Work out the finished part from the listing and answer in its coordinate system (mm). Round coordinates to 2 decimals unless told otherwise and drop trailing zeros. Loops run counter-clockwise (first coordinate to the right, second up) from the corner with the lowest first, then second, coordinate; pieces in that order, holes last. Notation, with made-up numbers: (5, 4.5) - (39, 4.5) arc R16 ccw to (39, 26.5) - close; hole circle Ø10 at (78.25, -4). An arc over 180 degrees is marked (long way). Return JSON: item names as keys, results as strings.
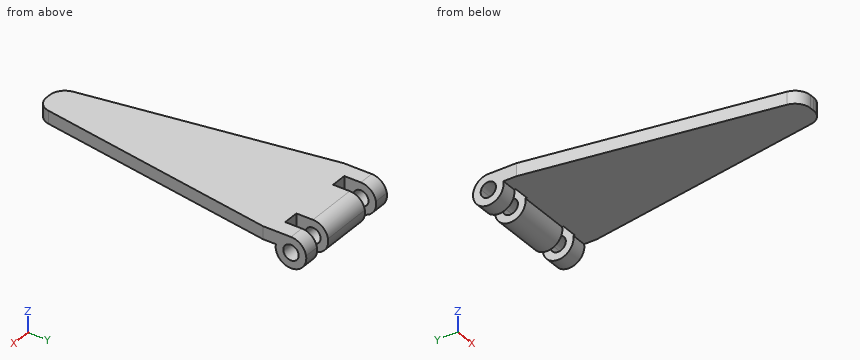
from build123d import *

# Parameters (mm, degrees)
CROQUIS1_W              = 45
CROQUIS1_H              = 17
SALIENTE_EXTRUIR1_DEPTH = 5
CROQUIS2_R              = 6
CROQUIS2_R_2            = 3
SALIENTE_EXTRUIR2_DEPTH = 45
CORTAR_EXTRUIR1_DEPTH   = 47.32763754
CROQUIS4_W              = 6.2
CROQUIS4_H              = 6.5
CROQUIS4_H_2            = 6
CORTAR_EXTRUIR2_DEPTH   = 27.879360111
SALIENTE_EXTRUIR3_DEPTH = 5
REDONDEO1_R             = 5.99


with BuildPart() as part:
    # Croquis1 → Saliente-Extruir1 (new body)
    with BuildSketch(Plane.XY):
        Rectangle(CROQUIS1_W, CROQUIS1_H)
    extrude(amount=SALIENTE_EXTRUIR1_DEPTH)

    # Croquis2 → Saliente-Extruir2 (add, through all)
    with BuildSketch(Plane(origin=(22.5, 0, 0), x_dir=(0, 0, -1), z_dir=(1, 0, 0))):
        with Locations((1, 2.5)):
            Circle(CROQUIS2_R)
        with Locations((1, 2.5)):
            Circle(CROQUIS2_R_2, mode=Mode.SUBTRACT)
    extrude(amount=-SALIENTE_EXTRUIR2_DEPTH)

    # Croquis3 → Cortar-Extruir1 (cut, through all)
    with BuildSketch(Plane(origin=(22.5, 0, 0), x_dir=(0, 0, -1), z_dir=(1, 0, 0))):
        with BuildLine():
            Line((-5, 8.5), (-5, 2.5))
            ThreePointArc((-5, 2.5), (-3.582575695, 6.372983346), (0, 8.416079783))
            Line((0, 8.416079783), (0, 8.5))
            Line((0, 8.5), (-5, 8.5))
        make_face()
        with BuildLine():
            ThreePointArc((0, -0.328427125), (2.732050808, 0.050510257), (4, 2.5))
            ThreePointArc((4, 2.5), (2.732050808, 4.949489743), (0, 5.328427125))
            Line((0, 5.328427125), (0, -0.328427125))
        make_face()
        with BuildLine():
            Line((0, -0.328427125), (0, 5.328427125))
            ThreePointArc((0, 5.328427125), (-2, 2.5), (0, -0.328427125))
        make_face()
    extrude(amount=-CORTAR_EXTRUIR1_DEPTH, mode=Mode.SUBTRACT)

    # Croquis4 → Cortar-Extruir2 (cut, through all)
    with BuildSketch(Plane.XY.offset(5)):
        with Locations((-13.35, -0.75)):
            Rectangle(CROQUIS4_W, CROQUIS4_H)
        with Locations((-13.35, 5.5)):
            Rectangle(CROQUIS4_W, CROQUIS4_H_2)
        with Locations((13.35, 5.5)):
            Rectangle(CROQUIS4_W, CROQUIS4_H_2)
        with Locations((13.35, -0.75)):
            Rectangle(CROQUIS4_W, CROQUIS4_H)
    extrude(amount=-CORTAR_EXTRUIR2_DEPTH, mode=Mode.SUBTRACT)

    # Croquis5 → Saliente-Extruir3 (add)
    with BuildSketch(Plane(origin=(0, 0, 0), x_dir=(-1, 0, 0), z_dir=(0, 0, -1))):
        Polygon((22.5, -8.5), (-22.5, -8.5), (-6, -108.5), (6, -108.5), align=None)
    extrude(amount=-SALIENTE_EXTRUIR3_DEPTH)

    # Redondeo1
    redondeo1_edges = [part.edges().sort_by_distance(p)[0] for p in [
        (6, -108.5, 2.5),
        (-6, -108.5, 2.5),
    ]]
    fillet(redondeo1_edges, radius=REDONDEO1_R)


solid = part.part
1) Section A-A (z = -5.5) is taken. Give the vertices of the cut face in (x, y).
Verdict:
{"outline": "(-22.5, -1.47) - (-16.45, -1.47) - (-16.45, 6.47) - (-22.5, 6.47) - close; (-10.25, -1.47) - (10.25, -1.47) - (10.25, 6.47) - (-10.25, 6.47) - close; (16.45, -1.47) - (22.5, -1.47) - (22.5, 6.47) - (16.45, 6.47) - close"}
2) Section D-D (y = -79) is taken. Give the vertices of the cut face in (x, z), and give its area (3 significant figures).
Verdict:
{"outline": "(-10.87, 0) - (10.87, 0) - (10.87, 5) - (-10.87, 5) - close", "area": "109 mm2"}
3) Section B-B (x = 17.5) is taken. Give the vertices of the cut face in (y, z).
Verdict:
{"outline": "(-38.8, 0) - (-3.42, 0) arc R6 ccw (long way) to (2.5, 5) - (-38.8, 5) - close; hole circle Ø6 at (2.5, -1)"}
4) Flat-ended cylindrical pins translate along their axes: pin 1 (5 mm diameter, centred on y = 2.5, z = -1, fed in from +X); pin 2 (12 mm diameter, centred on x = 11, y = -82, fed in from -Z); pin 3 (4 mm diameter, centred on y = -24.5, z = 3.5, fed in from -X); pin 4 (2.5 mm diameter, centred on x = -12.5, z = 2, fed in from +Y). Find the tip coordinate at first contact, or state that the pin passes through.
Verdict:
{"pin 1": "passes through", "pin 2": "stops at z = 0", "pin 3": "stops at x = -20.19", "pin 4": "stops at y = -4"}
5) Find the intervals of material crossed by L1, parallel to X at y = 0, z = 4.5; L2, parallel to Y at x = -18.75, z = -1; L3, parallel to Z at x = -0.5, y = 2.5, in increasing order.
Verdict:
{"L1": "x = -22.5 to -16.45, -10.25 to 10.25, 16.45 to 22.5", "L2": "y = -3.5 to -0.5, 5.5 to 8.5", "L3": "z = -7 to -4, 2 to 5"}
6) Section C-C (x = -18) is taken. Give the vertices of the cut face in (y, z), and give its area (3 significant figures).
Verdict:
{"outline": "(-35.77, 0) - (-3.42, 0) arc R6 ccw (long way) to (2.5, 5) - (-35.77, 5) - close; hole circle Ø6 at (2.5, -1)", "area": "254 mm2"}
